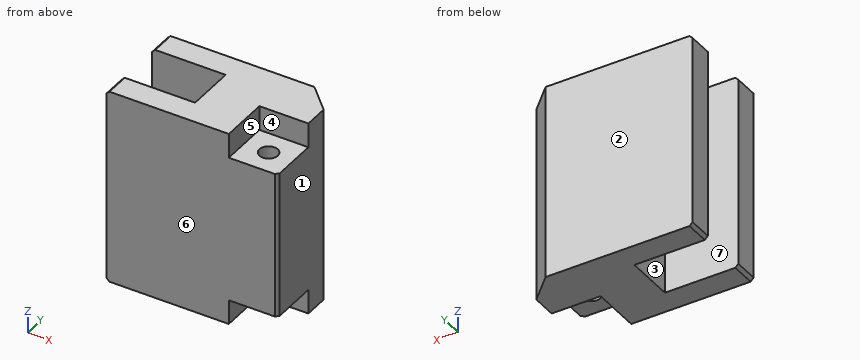
```python
from build123d import *

# Parameters (mm, degrees)
SKETCH1_W           = 88.9
SKETCH1_H           = 50.8
BOSS_EXTRUDE1_DEPTH = 50.8
SKETCH2_W           = 25.4
SKETCH2_H           = 25.4
CUT_EXTRUDE1_DEPTH  = 12.7
SKETCH3_R           = 4.7625
CUT_EXTRUDE2_DEPTH  = 103.587389576
SKETCH4_W           = 38.1
SKETCH4_H           = 25.4
CUT_EXTRUDE3_DEPTH  = 114.769602707
CHAMFER1_SIZE       = 12.7
CHAMFER2_SIZE       = 1.5875


with BuildPart() as part:
    # Sketch1 → Boss-Extrude1 (new, symmetric)
    with BuildSketch(Plane.XY):
        Rectangle(SKETCH1_W, SKETCH1_H)
    extrude(amount=BOSS_EXTRUDE1_DEPTH, both=True)

    # Sketch2 → Cut-Extrude1 (cut)
    with BuildSketch(Plane.XY.offset(50.8)):
        with Locations((31.75, -12.7)):
            Rectangle(SKETCH2_W, SKETCH2_H)
    cut_extrude1 = extrude(amount=-CUT_EXTRUDE1_DEPTH, mode=Mode.SUBTRACT)

    # Sketch3 → Cut-Extrude2 (cut, through all)
    with BuildSketch(Plane.XY.offset(38.1)):
        with Locations((31.75, -12.7)):
            Circle(SKETCH3_R)
    extrude(amount=-CUT_EXTRUDE2_DEPTH, mode=Mode.SUBTRACT)

    # Mirror1: Cut-Extrude1 across plane
    add(cut_extrude1.mirror(Plane.XY), mode=Mode.SUBTRACT)

    # Sketch4 → Cut-Extrude3 (cut, through all)
    with BuildSketch(Plane.XY.offset(50.8)):
        with Locations((-25.4, 0)):
            Rectangle(SKETCH4_W, SKETCH4_H)
    extrude(amount=-CUT_EXTRUDE3_DEPTH, mode=Mode.SUBTRACT)

    # Chamfer1
    chamfer1_edges = [part.edges().sort_by_distance(p)[0] for p in [
        (44.45, 25.4, 0),
    ]]
    chamfer(chamfer1_edges, length=CHAMFER1_SIZE)

    # Chamfer2
    chamfer2_edges = [part.edges().sort_by_distance(p)[0] for p in [
        (44.45, -25.4, 0),
        (-44.45, 19.05, 50.8),
        (-44.45, -19.05, 50.8),
        (-44.45, -19.05, -50.8),
        (-44.45, 19.05, -50.8),
    ]]
    chamfer(chamfer2_edges, length=CHAMFER2_SIZE)


solid = part.part
```
Check sheet for the modelled part. Datum: model origin and axes. Units: mm. Face numbers are marked on the shaded views. A direction names the side the tool comes from. Round coordinates to 2 decimals unless told otherwise and drop trailing zeros. Write each loop counter-clockwise with the first axis right and the second up, starting at its lowest first coordinate (ties: lowest second). Pieces come first, ordered by that corner, then holes. Notation, with made-up numbers: (27.5, 62) -> (61.5, 62) arc R19 cw to (61.5, 82) -> close; hole circle Ø9 at (38, 77). An arc over 180 degrees is marked (long way). One line per question, with ' | ' between items. Start each with the question number.
1. Sectioned sample at C-C, the plane y = 16.5. Record the cut outline in (x, z).
2. Scan lines: line 1 along Y through (x, z) = (31.75, 4.5); line 2 along X through (y, z) = (-13, 26.5); line 3 along X through (y, z) = (3, 15). Record each from-to range of solid material in increasing order. Write a range as from..to.
3. Release check for a two-part mould opening along Y. For the marked faces 1, 2, 3 and 4 record: +Y half, -Y half, draft (parallel to the pull), parting line (faces both ways), or undercut.
4. Depth check by flat-ended pin: pin 1 (12.5 mm diameter, centred on x = 35.5, y = -10, fed in from -Z); pin 2 (12.5 mm diameter, centred on y = -2.5, z = -18.5, fed in from -X); pin 3 (6.5 mm diameter, centred on y = -16, z = 45.5, fed in from +X); pin 4 (8.5 mm diameter, centred on x = 31.75, y = -12.7, fed in from +Z). Enter the tip coordinate at first touch or a pass-through.
5. Sectioned sample at D-D, the plane x = 39. Record the cut outline in (y, z).
6. Sectioned sample at B-B, the plane x = 25.5. Record the cut outline in (y, z).
7. Set-up check for the marked faces 5, 6 and 7: record each of +Z, -Z, +X, -X, +Y, -Y from which the full face is reachable in a straight line by a thin tool's end or side.
Taken from the geometry:
1) outline: (-44.45, -49.21) -> (-42.86, -50.8) -> (40.65, -50.8) -> (40.65, 50.8) -> (-42.86, 50.8) -> (-44.45, 49.21) -> close
2) line 1: y = -25.4..-17.46, -7.94..25.4 | line 2: x = -44.45..27, 36.5..44.45 | line 3: x = -6.35..44.45
3) face 1: draft | face 2: +Y half | face 3: undercut | face 4: -Y half
4) pin 1: stops at z = -38.1 | pin 2: stops at x = -6.35 | pin 3: stops at x = 19.05 | pin 4: passes through
5) outline: (-25.4, -38.1) -> (0, -38.1) -> (0, -50.8) -> (18.15, -50.8) -> (18.15, 50.8) -> (0, 50.8) -> (0, 38.1) -> (-25.4, 38.1) -> close
6) outline: (-25.4, -38.1) -> (0, -38.1) -> (0, -50.8) -> (25.4, -50.8) -> (25.4, 50.8) -> (0, 50.8) -> (0, 38.1) -> (-25.4, 38.1) -> close
7) face 5: +Z, +X, -Y | face 6: +Z, -Z, +X, -X, -Y | face 7: +Z, -Z, -X
